Autodesk Inventor part; units mm, degrees
ref_plane "YZ Plane" through (0, 0, 0) normal (1, 0, 0) x (0, 1, 0)
ref_plane "XZ Plane" through (0, 0, 0) normal (0, 1, 0) x (-1, 0, 0)
ref_plane "XY Plane" through (0, 0, 0) normal (0, 0, 1) x (1, 0, 0)
sketch "Sketch1" plane through (0, 0, 0) normal (0, 0, 1) x (1, 0, 0)
  line L0 (0, 40) -> (55.8, 40)
  line L1 (55.8, 40) -> (55.8, 0)
  line L2 (55.8, 0) -> (0, 0)
  line L3 (0, 0) -> (0, 40)
  dimension "d0" = 55.8
  dimension "d1" = 40
extrude "Extrusion1" add sketch "Sketch1" along normal blind 20
sketch "Sketch2" plane through (55.8, 0, 0) normal (1, 0, 0) x (0, 0, -1)
  line L0 (0, 40) -> (-20, 40)
  line L1 (0, 0) -> (0, 40)
  line L2 (-10, 40) -> (0, 40)
  line L3 (0, 40) -> (0, 12)
  line L4 (0, 12) -> (-10, 12)
  line L5 (-10, 12) -> (-10, 40)
  dimension "d4" = 10
extrude "Extrusion2" cut sketch "Sketch2" against normal blind 60
sketch "Sketch3" plane through (55.8, 12, 10) normal (0, 1, 0) x (1, 0, 0)
  circle A0 centre (-51.8, 4.52) radius 1.36
  circle A1 centre (-4, 4.52) radius 1.36
  line L0 (-55.8, 10) -> (0, 10)
  line L1 (-55.8, 0) -> (-55.8, 10)
  line L2 (0, 10) -> (0, 0)
  point P0 (-55.8, 5)
  point P1 (0, 5)
  dimension "d32" = 4
  dimension "d33" = 4
extrude "Extrusion3" cut sketch "Sketch3" against normal blind 20
sketch "Sketch4" plane through (0, 0, 20) normal (0, 0, 1) x (1, 0, 0)
  point P0 (0, 0)
sketch "Sketch6" plane through (0, 0, 0) normal (0, 0, -1) x (-1, 0, 0)
  circle A0 centre (-28, 20) radius 17.9
  point P0 (0, 0)
  dimension "d18" = 35.8
extrude "Extrusion4" cut sketch "Sketch6" along normal mid plane 60
sketch "Sketch8" plane through (0, 0, 0) normal (0, -1, 0) x (1, 0, 0)
  line L0 (49, 0) -> (6.8, 0)
  line L1 (6.8, 0) -> (6.8, 8)
  line L2 (6.8, 8) -> (49, 8)
  line L3 (49, 8) -> (49, 0)
  line L4 (55.8, 0) -> (55.8, 20)
  line L5 (0, 0) -> (0, 20)
  point P0 (6.8, 4)
  dimension "d27" = 6.8
  dimension "d28" = 6.8
extrude "Extrusion6" cut sketch "Sketch8" against normal blind 13
sketch "Sketch9" plane through (0, 0, 20) normal (0, -1, 0) x (1, 0, 0)
  line L0 (55.8, 0) -> (0, 0)
  line L1 (55.8, -10) -> (55.8, 0)
  line L2 (0, 0) -> (55.8, 0)
  line L3 (55.8, 0) -> (55.8, -10)
  line L4 (55.8, -10) -> (0, -10)
  line L5 (0, -10) -> (0, 0)
  point P0 (0, -20)
  dimension "d34" = 10
extrude "Extrusion7" add sketch "Sketch9" along normal blind 30
sketch "Sketch10" plane through (0, -30, 20) normal (0, -1, 0) x (1, 0, 0)
  line L0 (0, -10) -> (0, 0)
  line L1 (55.8, -10) -> (55.8, 0)
  line L2 (0, -2) -> (55.8, -2)
  line L3 (55.8, -2) -> (55.8, -6)
  line L4 (55.8, -6) -> (0, -6)
  line L5 (0, -6) -> (0, -2)
  point P0 (0, -20)
  point P1 (0, -6)
extrude "Extrusion8" cut sketch "Sketch10" against normal blind 20
Source: CAD feature listing. Evaluate the final solid. Frame: model axes, mm. A direction names the side the tool comes from. Give positions to 0.01 mm unless a question says otherwise; leave off trailing zeros. Write each loop counter-clockwise with the first axis right and the second up, starting at its lowest first coordinate (ties: lowest second). Pieces come first, ordered by that corner, then holes. Notation, with made-up numbers: (-5.5, 87) - (20.5, 87) arc R31 cw to (20.5, 116) - close; hole circle Ø11 at (44, -5). An arc over 180 degrees is marked (long way). One line per item, written item: value. Start each with the question number.
Q1. First-contact query: pin 1 Ø4.5 at (x, z) = (4, 5.48) entering from +Y; pin 2 Ø8 at (x, z) = (46, 9.5) entering from -Y; pin 3 Ø2 at (x, z) = (25.5, 16.5) entering from -Y; pin 4 Ø14 at (x, y) = (24.5, 28.5) entering from -Z. Flat tips, straight axial feed; report the tip coordinate or a pass-through.
Q2. Material intervals for probe 1 along X at (y, z) = (7.5, 5.48); probe 2 along Y at (x, z) = (28, 12.5); probe 3 along X at (y, z) = (20, 12.5), sorted ascending. Write a range as from..to.
Q3. Set-up query: faces 5 (the face through (31.88, 2.526, 15.249)), 6 (the face through (28, -15, 10)), 7 (the face through (49, 6, 4)), 8 (the face through (5, 12, 7)). Return all of +Z, -Z, +X, -X, +Y, -Y with unobstructed straight access to the full face (end or side cutting, diameter ignored); none if empty.
Q4. Section query B-B, the plane y = 20. Return the cut outline in (x, z), then the cut area to 3 significant figures.
Q5. Section query C-C, the plane x = 4. Return the cut outline in (y, z), then the cut area to 3 significant figures.
Q6. Section query A-A, the plane z = 2.25. Return the cut outline in (x, y).
Q7. Draft query along Z for faces 1 (the face through (2.921, 6.084, 6.308)), 2 (the face through (6.8, 6, 4)), 3 (the face through (28.3, 38.2, 10)), 4 (the face through (28, -10, 16)). Return one class per face: +Z half, -Z half, draft (parallel to the pull), parting line (faces both ways), or undercut.
Q8. Section query D-D, the plane y = 1. Return the cut outline in (x, z), then the cut area to 3 significant figures.
Answer:
1. pin 1: stops at y = 12
1. pin 2: stops at y = -30
1. pin 3: stops at y = -10
1. pin 4: passes through
2. probe 1: x = 0..2.64, 5.36..6.8, 49..50.44, 53.16..55.8
2. probe 2: y = -30..2.1, 37.9..40
2. probe 3: x = 0..10.1, 45.9..55.8
3. face 5: +Z, -Z
3. face 6: -Z, +X, -X, -Y
3. face 7: -Z, +Y, -Y
3. face 8: -Z, +X, -X, +Y
4. outline: (0, 10) - (10.1, 10) - (10.1, 20) - (0, 20) - close; (45.9, 10) - (55.8, 10) - (55.8, 20) - (45.9, 20) - close
4. area: 200 mm2
5. outline: (-30, 10) - (0, 10) - (0, 6.84) - (12, 6.84) - (12, 10) - (40, 10) - (40, 20) - (-30, 20) - (-30, 18) - (-10, 18) - (-10, 14) - (-30, 14) - close; (0, 0) - (12, 0) - (12, 4.12) - (0, 4.12) - close
5. area: 707 mm2
6. outline: (0, 0) - (6.8, 0) - (6.8, 12) - (0, 12) - close; (49, 0) - (55.8, 0) - (55.8, 12) - (49, 12) - close
7. face 1: undercut
7. face 2: draft
7. face 3: -Z half
7. face 4: undercut
8. outline: (0, 0) - (6.8, 0) - (6.8, 8) - (49, 8) - (49, 0) - (55.8, 0) - (55.8, 20) - (0, 20) - close; hole circle Ø2.72 at (4, 5.48); hole circle Ø2.72 at (51.8, 5.48)
8. area: 767 mm2
